Drawing for the job (mm, zero at the part's lowest x, y, z). A direction names the side the tool comes from. Give positions to 0.01 mm unless a question says otherwise; leave off trailing zeros. Write each loop counter-clockwise with the first axis right and the second up, starting at its lowest first coordinate (ties: lowest second). Pieces come first, ordered by that corner, then holes. Notation, with made-up numbers: M -33,-7.5 L -9,-7.5 A22 ccw -9,15.5 Z; hole C 57.5,-1 d7. An arc over 180 degrees is marked long. Write item = value, one per line. Start each with the question number.
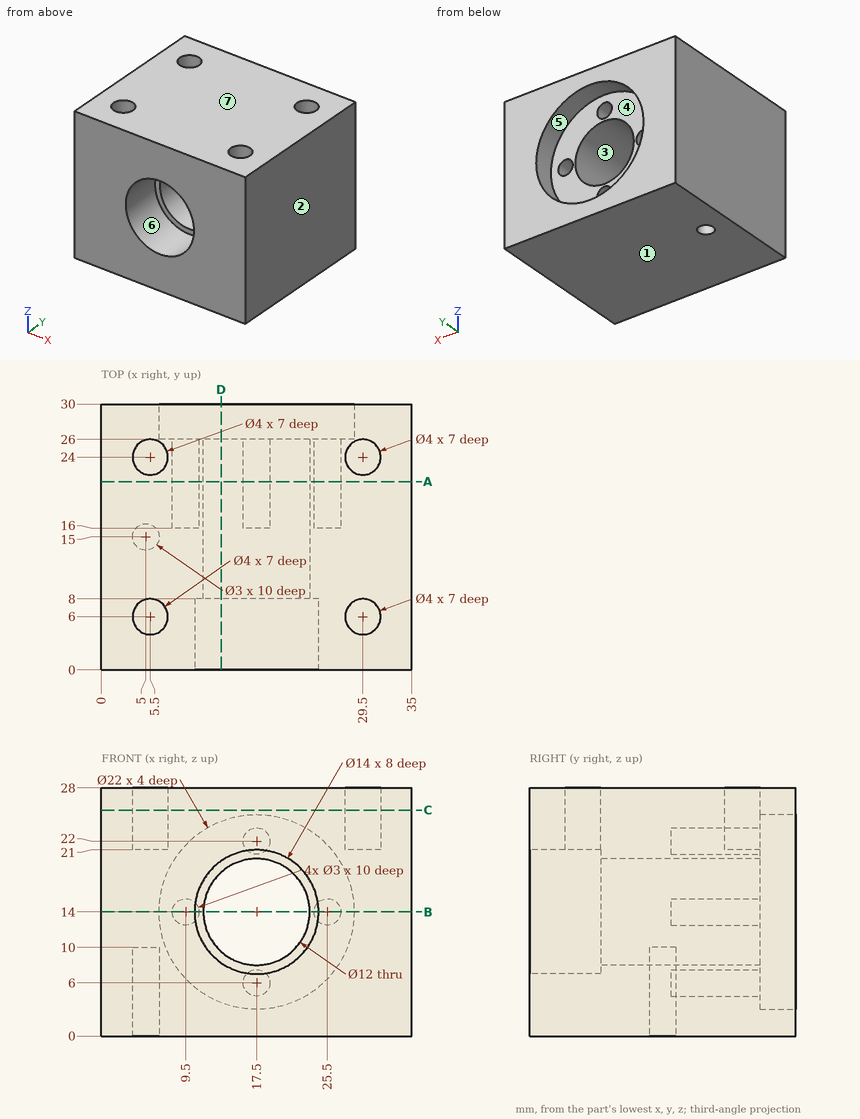
Q1. Two-plate mould, pull along Z, no slides. Class the marked faces 1, 2, 3 and 4: +Z half, -Z half, draft (parallel to the pull), parting line (faces both ways), or undercut.
Q2. Tool access for the marked faces 5, 6 and 7: list every direction of +Z, -Z, +X, -X, +Y, -Y with a clear straight run to the whole face (end or side of a thin tool).
Q3. Slice it at B-B (z = 14). Give the cut face in (x, y), and give its area (3 significant figures).
Q4. Slice it at C-C (z = 25.5). Give the cut face in (x, y), and give its area (4 significant figures).
Q5. Drop flat-ended pins along their axis: P1, Ø8, axis at y = 19.5, z = 12.5, coming from the -X side; P2, Ø1.5, axis at x = 18, z = 6.5, coming from the +Y side; P3, Ø7, axis at x = 19, z = 14, coming from the -Y side; P4, Ø2.5, axis at x = 25.5, z = 14.5, coming from the +Y side. Give the stop position or say it passes through.
Q6. Probe line 1 along Z through (x, y) = (17.5, 19.25); line 2 along Y through (x, z) = (29.5, 23.25); line 3 along Y through (x, z) = (5, 3.5). List the from-to ranges inside material, lowest first.
Q7. Slice it at A-A (y = 21.25). Give the cut face in (x, z), and give its area (3 significant figures).
Q8. Slice it at D-D (x = 13.5). Give the cut face in (y, z).
Working result:
q1.face_1 = -Z half
q1.face_2 = draft
q1.face_3 = undercut
q1.face_4 = undercut
q2.face_5 = +Y
q2.face_6 = -Y
q2.face_7 = +Z, +X, -X, +Y, -Y
q3.outline = M 0,0 L 10.5,0 L 10.5,8 L 11.5,8 L 11.5,26 L 11,26 L 11,16 L 8,16 L 8,26 L 6.5,26 L 6.5,30 L 0,30 Z; M 23.5,8 L 24.5,8 L 24.5,0 L 35,0 L 35,30 L 28.5,30 L 28.5,26 L 27,26 L 27,16 L 24,16 L 24,26 L 23.5,26 Z
q3.area = 574 mm2
q4.outline = M 0,0 L 35,0 L 35,30 L 0,30 Z; hole C 5.5,6 d4; hole C 5.5,24 d4; hole C 29.5,6 d4; hole C 29.5,24 d4
q4.area = 1,000 mm2
q5.P1 = 0
q5.P2 = 16
q5.P3 = through
q5.P4 = 26
q6.line_1 = 0 to 4.5, 7.5 to 8, 20 to 20.5, 23.5 to 28
q6.line_2 = 0 to 4, 8 to 22, 26 to 30
q6.line_3 = 0 to 13.5, 16.5 to 30
q7.outline = M 0,0 L 35,0 L 35,28 L 0,28 Z; hole C 9.5,14 d3; hole C 17.5,14 d12; hole C 17.5,6 d3; hole C 17.5,22 d3; hole C 25.5,14 d3
q7.area = 839 mm2
q8.outline = M 0,0 L 30,0 L 30,3.75 L 26,3.75 L 26,9.53 L 8,9.53 L 8,8.26 L 0,8.26 Z; M 0,19.74 L 8,19.74 L 8,18.47 L 26,18.47 L 26,24.25 L 30,24.25 L 30,28 L 0,28 Z
